Source: CAD feature listing. Evaluate the final solid. Frame: model axes, mm. Face numbers are marked on the shaded views. A direction names the side the tool comes from. Give positions to 0.01 mm unless a question says otherwise; leave off trailing zeros. Write each loop counter-clockwise with the first axis right and the second up, starting at its lowest first coordinate (ties: lowest second). Pieces come first, ordered by that corner, then holes. Notation, with made-up numbers: (52.25, 71) -> (76.25, 71) arc R25 ccw to (76.25, 92) -> close; hole circle Ø7 at (-12.75, 78.25). An arc over 180 degrees is marked (long way). Use one line per item in the form item = value. Start each with the question number.
(1) Cut plane C-C, the plane x = 199. Output: boundary loops of the cut face in (y, z).
(2) First-contact query: P1, Ø3, axis at x = 177, z = 3, coming from the +Y side; P2, Ø2, axis at x = 177.5, y = -19.5, coming from the +Z side; P3, Ø0.8, axis at x = 184, z = 1, coming from the -Y side. Flat tips, straight axial feed; report the tip coordinate or a pass-through.
(3) Cut plane B-B, the plane y = -3. Output: boundary loops of the cut face in (x, z).
(4) Draft query along X for the marked faces 4, 5 and 6. Return one class per face: pulls with the +X half, pulls with the -X half, needs draft (parallel to the pull), parting line crosses it, or undercut.
(5) Cut plane A-A, the plane z = 4.75. Output: boundary loops of the cut face in (x, y).
(6) Set-up query: the marked faces 1, 2 and 3. Return all of +Z, -Z, +X, -X, +Y, -Y with unobstructed straight access to the full face (end or side cutting, diameter ignored); none if empty.
(7) Material intervals for line 1 along Y through (x, z) = (150.5, 6.5); line 2 along Z through (x, y) = (132, -2); line 3 along X through (y, z) = (-19, 4), sorted ascending. Write a range as from..to.
(8) Cut plane D-D, the plane z = -1.5. Output: boundary loops of the cut face in (x, y), and give its area (3 significant figures).
from build123d import *

# Parameters (mm, degrees)
SKETCH048_W     = 70.5
SKETCH048_H     = 25.7
PAD041_DEPTH    = 9.5
THICKNESS005_T  = 2.5
SKETCH049_R     = 3
POCKET011_DEPTH = 2.5
SKETCH050_W     = 70.5
SKETCH050_H     = 1.5
PAD042_DEPTH    = 2.5
PAD040_DEPTH    = 2.5


with BuildPart() as body014:
    # Sketch048 → Pad041 (new body)
    with BuildSketch(Plane.XY):
        with Locations((0, -48)):
            Rectangle(SKETCH048_W, SKETCH048_H)
    extrude(amount=PAD041_DEPTH)

    # Thickness005
    thickness005_openings = [body014.faces().sort_by_distance(p)[0] for p in [
        (0, -48, 9.5),
        (0, -48, 0),
    ]]
    offset(amount=THICKNESS005_T, openings=thickness005_openings, kind=Kind.INTERSECTION)

    # Sketch049 (on Face6 of Thickness005) → Pocket011 (cut)
    with BuildSketch(Plane(origin=(-37.75, 0, 0), x_dir=(0, -1, 0), z_dir=(-1, 0, 0))):
        with Locations((39, 4.75)):
            Circle(SKETCH049_R)
    extrude(amount=-POCKET011_DEPTH, mode=Mode.SUBTRACT)

    # Sketch050 → Pad042 (join)
    with BuildSketch(Plane.XY):
        with Locations((0, -35.75)):
            Rectangle(SKETCH050_W, SKETCH050_H)
    extrude(amount=PAD042_DEPTH)


with BuildPart() as body014_1:
    # Body014 placement: moved
    add(body014.part.moved(Location((84.5, 36.85, 0))))


with BuildPart() as tail:
    # Sketch047 → Pad040 (new body)
    with BuildSketch(Plane(origin=(0, 0, 0), x_dir=(1, 0, 0), z_dir=(0, 0, -1))):
        with BuildLine():
            Line((-40.250166, 30.15), (37.1, 30.15))
            ThreePointArc((37.1, 30.15), (38.867767, 30.882233), (39.6, 32.65))
            Line((39.6, 63.35), (39.6, 32.65))
            ThreePointArc((39.6, 63.35), (38.867767, 65.117767), (37.1, 65.85))
            Line((37.1, 65.85), (-40.25, 65.85))
            Line((-40.25, 65.85), (-40.25, 59.35))
            Line((-40.25, 59.35), (-44.1, 61.572799))
            Line((-44.1, 61.572799), (-44.1, 51.292346))
            Line((-44.1, 51.292346), (-40.25, 53.515144))
            Line((-40.25, 53.515144), (-40.25, 42.485144))
            Line((-40.25, 42.485144), (-44.100166, 44.707654))
            Line((-44.100166, 44.707654), (-44.100166, 34.427201))
            Line((-44.100166, 34.427201), (-40.250166, 36.65))
            Line((-40.250166, 36.65), (-40.250166, 30.15))
        make_face()
    extrude(amount=PAD040_DEPTH)


with BuildPart() as tail_1:
    # Body013 placement: moved
    add(tail.part.moved(Location((84.5, 36.85, 0))))

    # Fusion004: union Body014
    add(body014_1.part)


with BuildPart() as tail_2:
    # Fusion004 placement: moved
    add(tail_1.part.moved(Location((84.5, 0, 0))))


solid = tail_2.part
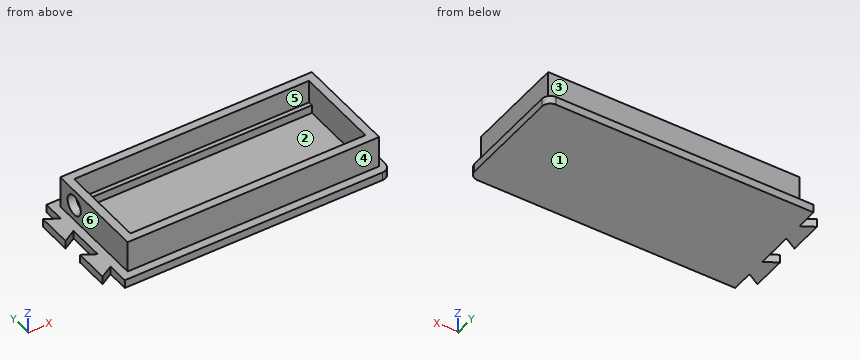
Geometry says:
q1.outline = (-29, -2.5) -> (6.7, -2.5) -> (6.7, 0) -> (4.2, 0) -> (4.2, 9.5) -> (1.7, 9.5) -> (1.7, 2.5) -> (0.35, 2.5) -> (0.35, 0) -> (-24, 0) -> (-24, 9.5) -> (-26.5, 9.5) -> (-26.5, 0) -> (-29, 0) -> close
q2.P1 = 4.2
q2.P2 = 0
q2.P3 = -26.5
q3.outline = (124.9, -2.5) -> (208.6, -2.5) -> (208.6, 0) -> (206.75, 0) -> (206.75, 9.5) -> (204.25, 9.5) -> (204.25, 0) -> (133.75, 0) -> (133.75, 1.87) -> (131.25, 1.87) -> (131.25, 0) -> (124.9, 0) -> close; (131.25, 7.63) -> (133.75, 7.63) -> (133.75, 9.5) -> (131.25, 9.5) -> close
q4.face_4 = needs draft
q4.face_5 = undercut
q4.face_6 = pulls with the -X half
q5.outline = (131.25, -26.5) -> (206.75, -26.5) -> (206.75, 4.2) -> (131.25, 4.2) -> (131.25, 0.85) -> (133.75, 0.85) -> (133.75, 1.7) -> (204.25, 1.7) -> (204.25, -24) -> (133.75, -24) -> (133.75, -5.15) -> (131.25, -5.15) -> close
q6.face_1 = -Z, +X, -X, +Y, -Y
q6.face_2 = +Z
q6.face_3 = +Z, +X, -X, +Y
q7.line_1 = -26.5..-24, 1.7..4.2
q7.line_2 = -2.5..1.75, 7.75..9.5
q7.line_3 = 131.25..133.75, 204.25..206.75
q8.outline = (124.9, -24.72) -> (128.75, -22.5) -> (128.75, -29) -> (206.1, -29) arc R2.5 ccw to (208.6, -26.5) -> (208.6, 4.2) arc R2.5 ccw to (206.1, 6.7) -> (128.75, 6.7) -> (128.75, 0.2) -> (124.9, 2.42) -> (124.9, -7.86) -> (128.75, -5.64) -> (128.75, -16.67) -> (124.9, -14.44) -> close
q8.area = 2,910 mm^2
